from build123d import *

# Parameters (mm, degrees)
SKETCH1_W           = 50
SKETCH1_H           = 50
SKETCH1_R           = 8
SKETCH1_R_2         = 1.6
SKETCH1_R_3         = 1.5
SKETCH1_R_4         = 1.4
BOSS_EXTRUDE1_DEPTH = 1.6
FILLET1_R           = 3


with BuildPart() as part:
    # Sketch1 → Boss-Extrude1 (new body)
    with BuildSketch(Plane(origin=(0, 0, 0), x_dir=(1, 0, 0), z_dir=(0, 1, 0))):
        Rectangle(SKETCH1_W, SKETCH1_H)
        with Locations(Location((0, 0, 0), (0, 0, 270))):
            Circle(SKETCH1_R, mode=Mode.SUBTRACT)
        with Locations(Location((-22.525126266, 22.525126266, 0), (0, 0, 270))):
            Circle(SKETCH1_R_2, mode=Mode.SUBTRACT)
        with Locations(Location((-17.575378798, 17.575378798, 0), (0, 0, 270))):
            Circle(SKETCH1_R_3, mode=Mode.SUBTRACT)
        with Locations(Location((-4, 22, 0), (0, 0, 270))):
            Circle(SKETCH1_R_4, mode=Mode.SUBTRACT)
        with Locations(Location((-11.5, 22, 0), (0, 0, 270))):
            Circle(SKETCH1_R_4, mode=Mode.SUBTRACT)
        with Locations(Location((4, 22, 0), (0, 0, 90))):
            Circle(SKETCH1_R_4, mode=Mode.SUBTRACT)
        with Locations(Location((11.5, 22, 0), (0, 0, 90))):
            Circle(SKETCH1_R_4, mode=Mode.SUBTRACT)
        with Locations(Location((22, 11.5, 0), (0, 0, 270))):
            Circle(SKETCH1_R_4, mode=Mode.SUBTRACT)
        with Locations(Location((22, 4, 0), (0, 0, 270))):
            Circle(SKETCH1_R_4, mode=Mode.SUBTRACT)
        with Locations(Location((22, -4, 0), (0, 0, 90))):
            Circle(SKETCH1_R_4, mode=Mode.SUBTRACT)
        with Locations(Location((22, -11.5, 0), (0, 0, 90))):
            Circle(SKETCH1_R_4, mode=Mode.SUBTRACT)
        with Locations(Location((11.5, -22, 0), (0, 0, 270))):
            Circle(SKETCH1_R_4, mode=Mode.SUBTRACT)
        with Locations(Location((4, -22, 0), (0, 0, 270))):
            Circle(SKETCH1_R_4, mode=Mode.SUBTRACT)
        with Locations(Location((-4, -22, 0), (0, 0, 90))):
            Circle(SKETCH1_R_4, mode=Mode.SUBTRACT)
        with Locations(Location((-11.5, -22, 0), (0, 0, 90))):
            Circle(SKETCH1_R_4, mode=Mode.SUBTRACT)
        with Locations(Location((-22, -11.5, 0), (0, 0, 270))):
            Circle(SKETCH1_R_4, mode=Mode.SUBTRACT)
        with Locations(Location((-22, -4, 0), (0, 0, 270))):
            Circle(SKETCH1_R_4, mode=Mode.SUBTRACT)
        with Locations(Location((-22, 4, 0), (0, 0, 90))):
            Circle(SKETCH1_R_4, mode=Mode.SUBTRACT)
        with Locations(Location((-22, 11.5, 0), (0, 0, 90))):
            Circle(SKETCH1_R_4, mode=Mode.SUBTRACT)
        with Locations(Location((22.525126266, 22.525126266, 0), (0, 0, 270))):
            Circle(SKETCH1_R_2, mode=Mode.SUBTRACT)
        with Locations(Location((17.575378798, 17.575378798, 0), (0, 0, 270))):
            Circle(SKETCH1_R_3, mode=Mode.SUBTRACT)
        with Locations(Location((22.525126266, -22.525126266, 0), (0, 0, 270))):
            Circle(SKETCH1_R_2, mode=Mode.SUBTRACT)
        with Locations(Location((17.575378798, -17.575378798, 0), (0, 0, 270))):
            Circle(SKETCH1_R_3, mode=Mode.SUBTRACT)
        with Locations(Location((-22.525126266, -22.525126266, 0), (0, 0, 270))):
            Circle(SKETCH1_R_2, mode=Mode.SUBTRACT)
        with Locations(Location((-17.575378798, -17.575378798, 0), (0, 0, 270))):
            Circle(SKETCH1_R_3, mode=Mode.SUBTRACT)
    extrude(amount=BOSS_EXTRUDE1_DEPTH)

    # Fillet1
    fillet1_edges = [part.edges().sort_by_distance(p)[0] for p in [
        (25, 0.8, 25),
        (-25, 0.8, 25),
        (-25, 0.8, -25),
        (25, 0.8, -25),
    ]]
    fillet(fillet1_edges, radius=FILLET1_R)


solid = part.part
The listing builds one solid part. Answer for the finished solid, in the listing's coordinates (mm). Round coordinates to 2 decimals unless told otherwise and drop trailing zeros. Write each loop counter-clockwise with the first axis right and the second up, starting at its lowest first coordinate (ties: lowest second). Pieces come first, ordered by that corner, then holes. Notation, with made-up numbers: M 16,87 L 35,87 A38 cw 35,125 Z; hole C 5.25,-33.5 d11. An arc over 180 degrees is marked long. Write each question's results on one line, items separated by ' | '. Start each with the question number.
Item 1: Find section B-B on x = 0. Write down the section's boundary in (y, z).
Item 2: The mould has two halves that part along X. Classify faces 1 (the cylindrical face through (24.1, 0.81, -24.14)), 2 (the flat face through (-25, 1, 0)), 3 (the cylindrical face through (23.61, 0.79, 21.35)): +X half, -X half, draft (parallel to the pull), parting line (faces both ways), or undercut.
Item 3: Find section A-A on z = -11.5. Write down the section's boundary in (x, y).
Item 4: Straight lines are drawn through the part: probe 1 along X at (y, z) = (1.25, 11.5); probe 2 along X at (y, z) = (0.3, -3); probe 3 along X at (y, z) = (1.3, 5.5). For each, find the intervals that lie inside material, in ascending order.
Item 5: Find section D-D on z = 0.5. Write down the section's boundary in (x, y), and give its area (4 significant figures).
Item 6: Find section C-C on x = 11.5. Write down the section's boundary in (y, z), and give its area (3 significant figures).
Answer block:
1) outline: M 0,-25 L 1.6,-25 L 1.6,-8 L 0,-8 Z; M 0,8 L 1.6,8 L 1.6,25 L 0,25 Z
2) face 1: +X half | face 2: -X half | face 3: undercut
3) outline: M -25,0 L -23.4,0 L -23.4,1.6 L -25,1.6 Z; M -20.6,0 L 20.6,0 L 20.6,1.6 L -20.6,1.6 Z; M 23.4,0 L 25,0 L 25,1.6 L 23.4,1.6 Z
4) probe 1: x = -25 to -23.4, -20.6 to 20.6, 23.4 to 25 | probe 2: x = -25 to -22.98, -21.02 to -7.42, 7.42 to 21.02, 22.98 to 25 | probe 3: x = -25 to -5.81, 5.81 to 25
5) outline: M -25,0 L -7.98,0 L -7.98,1.6 L -25,1.6 Z; M 7.98,0 L 25,0 L 25,1.6 L 7.98,1.6 Z | area: 54.45 mm²
6) outline: M 0,-25 L 1.6,-25 L 1.6,-23.4 L 0,-23.4 Z; M 0,-20.6 L 1.6,-20.6 L 1.6,20.6 L 0,20.6 Z; M 0,23.4 L 1.6,23.4 L 1.6,25 L 0,25 Z | area: 71.0 mm²
